```python
from build123d import *

# Parameters (mm, degrees)
F2_DEPTH = 5
F3_W     = 2
F3_H     = 2
F4_DEPTH = 150.001


# Not quite as in the source:
# - a feature names something its author has since deleted; it is built from what else it names


with BuildPart() as f2:
    # F1 (on Front) → F2 (new body)
    with BuildSketch(Plane.XZ):
        Polygon((70, -8), (70, 0), (-70, 0), (-70, -8), (-75, -8), (-75, -16), (-70, -16), (-70, -24), (-75, -24), (-75, -32), (-70, -32), (-70, -40), (-75, -40), (-75, -48), (-70, -48), (-70, -56), (-75, -56), (-75, -64), (-70, -64), (-70, -72), (-75, -72), (-75, -80), (75, -80), (75, -72), (70, -72), (70, -64), (75, -64), (75, -56), (70, -56), (70, -48), (75, -48), (75, -40), (70, -40), (70, -32), (75, -32), (75, -24), (70, -24), (70, -16), (75, -16), (75, -8), align=None)
    extrude(amount=F2_DEPTH)

    # F3 (on face) → F4 (cut, through all)
    with BuildSketch(Plane.YZ.offset(75)):
        with Locations((-1, -76)):
            Rectangle(F3_W, F3_H)
    extrude(amount=-F4_DEPTH, mode=Mode.SUBTRACT)


solid = f2.part
```
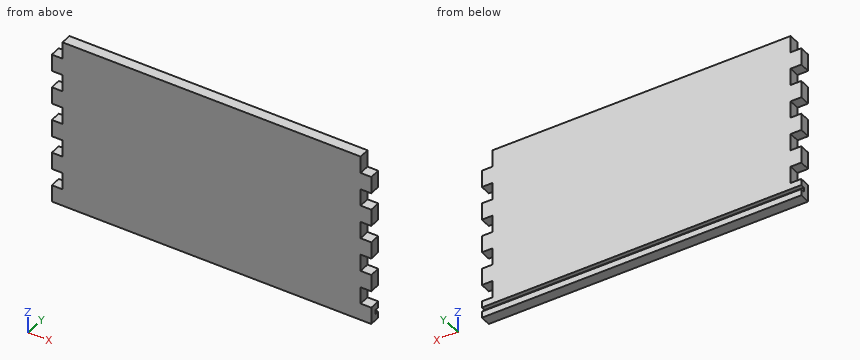
The model under review builds one solid part; all positions refer to its coordinate system, in mm. Round coordinates to 2 decimals unless told otherwise and drop trailing zeros. Order: outer loops, then holes, each group sorted by start corner. A loop starts at its lowest first (then second) coordinate and runs counter-clockwise, first axis right, second up. Notation, with made-up numbers: (24, 88.25) -> (71, 88.25) arc R19 ccw to (71, 97.25) -> close; hole circle Ø2 at (78.5, -0.5). An arc over 180 degrees is marked (long way). One line per item, written item: value. Start each with the question number.
Q1. Take a section at A-A (z = -20). Write out the cut boundary in (x, y).
Q2. Wall thickness on line 1 (Z direction, x = 26, y = -1.6); line 2 (X direction, y = -4.4, z = -64.5): over which ranges is each line inside the solid? List them lowest first.
Q3. Clearance check with flat-ended pins moving along their axes: pin 1 Ø1 at (y, z) = (-4.5, -19) entering from +X; pin 2 Ø2 at (x, z) = (11.5, -12.5) entering from +Y; pin 3 Ø2.5 at (y, z) = (-2, -53) entering from -X; pin 4 Ø1.5 at (x, y) = (73.5, -3.5) entering from +Z. State where each tip first meets the part, or that it passes through.
Reported:
1. outline: (-70, -5) -> (70, -5) -> (70, 0) -> (-70, 0) -> close
2. line 1: z = -80 to -77, -75 to 0
2. line 2: x = -70 to 70
3. pin 1: stops at x = 70
3. pin 2: stops at y = 0
3. pin 3: stops at x = -70
3. pin 4: stops at z = -8
